Here's the drawing with two shaded views (mm, measured from the low corner). I have some questions. A direction names the side the tool comes from. Coordinates: 2 decimals unless noted, no trailing zeros. Write each loop counter-clockwise with the first axis right and the second up, starting at its lowest first coordinate (ties: lowest second). Pieces come first, ordered by that corner, then holes. Notation, with made-up numbers: (79.25, 55.5) - (116.25, 55.5) arc R23 ccw to (116.25, 90.5) - close; hole circle Ø6 at (7.25, 60.25). An arc over 180 degrees is marked (long way). Answer in a Markdown table with one row per item. Add a question column.
Item 1: Imagine slicing it at B-B (y = 19.05). Please give me the cut outline in (x, z).
Item 2: Imagine slicing it at D-D (z = 30). Please give me the cut outline in (x, y), plus the area to 3 significant figures.
Item 3: We'd pull the mould along X, two halves only. Please class the marked faces 3, 4 and 5: +X half, -X half, draft (parallel to the pull), parting line (faces both ways), or undercut.
Item 4: Imagine slicing it at A-A (z = 57.15). Please give me the cut outline in (x, y).
Item 5: If I drill on probe 1 along Y at (x, z) = (19, 3); probe 2 along X at (y, z) = (33, 73), over which ranges is the centre line in solid material (lowest first)? Write a range as from..to.
Item 6: Imagine slicing it at C-C (x = 57.15). Please give me the cut outline in (y, z).
Item 7: I'm going to push a flat-ended pin straight in: pin 1 (1 mm diameter, centred on x = 44, y = 13, fed in from +Z). Where does the tip first touch, or does it pass through?
Item 8: Which directions (+Z, -Z, +X, -X, +Y, -Y) give clear straight access to the entire face, cutting with the end or side of a thin tool? Please do the marked faces 1 and 2.
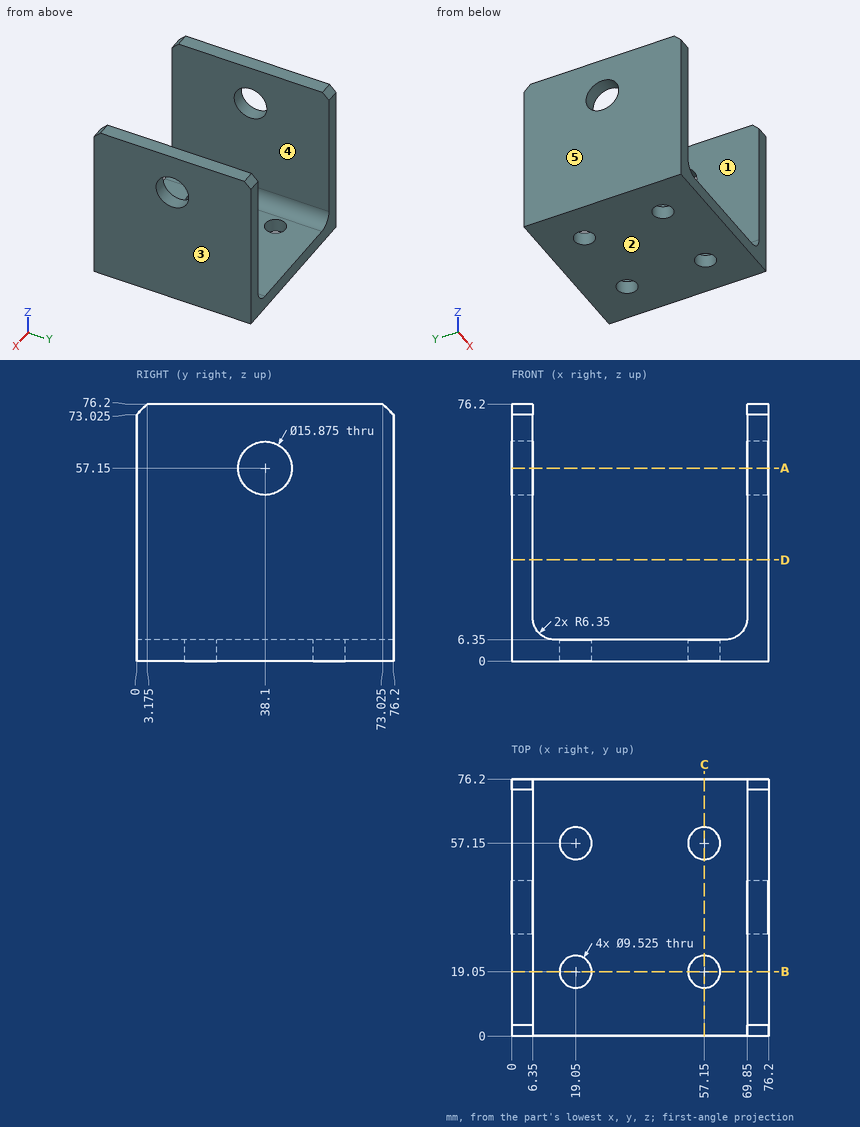
Here are the results:
| question | item | result |
|---|---|---|
| 1 | outline | (0, 0) - (14.29, 0) - (14.29, 6.35) - (12.7, 6.35) arc R6.35 cw to (6.35, 12.7) - (6.35, 76.2) - (0, 76.2) - close; (23.81, 0) - (52.39, 0) - (52.39, 6.35) - (23.81, 6.35) - close; (61.91, 0) - (76.2, 0) - (76.2, 76.2) - (69.85, 76.2) - (69.85, 12.7) arc R6.35 cw to (63.5, 6.35) - (61.91, 6.35) - close |
| 2 | outline | (0, 0) - (6.35, 0) - (6.35, 76.2) - (0, 76.2) - close; (69.85, 0) - (76.2, 0) - (76.2, 76.2) - (69.85, 76.2) - close |
| 2 | area | 968 mm2 |
| 3 | face 3 | +X half |
| 3 | face 4 | undercut |
| 3 | face 5 | -X half |
| 4 | outline | (0, 0) - (6.35, 0) - (6.35, 30.16) - (0, 30.16) - close; (0, 46.04) - (6.35, 46.04) - (6.35, 76.2) - (0, 76.2) - close; (69.85, 0) - (76.2, 0) - (76.2, 30.16) - (69.85, 30.16) - close; (69.85, 46.04) - (76.2, 46.04) - (76.2, 76.2) - (69.85, 76.2) - close |
| 5 | probe 1 | y = 0..14.29, 23.81..52.39, 61.91..76.2 |
| 5 | probe 2 | x = 0..6.35, 69.85..76.2 |
| 6 | outline | (0, 0) - (14.29, 0) - (14.29, 6.35) - (0, 6.35) - close; (23.81, 0) - (52.39, 0) - (52.39, 6.35) - (23.81, 6.35) - close; (61.91, 0) - (76.2, 0) - (76.2, 6.35) - (61.91, 6.35) - close |
| 7 | pin 1 | stops at z = 6.35 |
| 8 | face 1 | +Z, +Y, -Y |
| 8 | face 2 | -Z, +X, -X, +Y, -Y |
